CAD build for the part. Positions are in the model's coordinates, mm. Give positions to 0.01 mm unless a question says otherwise; leave off trailing zeros. Write each loop counter-clockwise with the first axis right and the second up, starting at its lowest first coordinate (ties: lowest second). Pieces come first, ordered by that corner, then holes. Notation, with made-up numbers: (-12, 38) - (6, 38) arc R18 ccw to (6, 56) - close; hole circle Ø7 at (-34, 54). An arc over 180 degrees is marked (long way). Write item = value, one per line. Start each with the question number.
```python
from build123d import *

# Parameters (mm, degrees)
F1_DEPTH = 1.6002
F3_DEPTH = 1.6012
F4_R     = 1.9939
F4_R_2   = 1.770589
F5_DEPTH = 1.6012


with BuildPart() as f1:
    # F0 (on Top) → F1 (new body)
    with BuildSketch(Plane.XY):
        with BuildLine():
            ThreePointArc((-241.3, -104.775), (-239.440128, -109.265128), (-234.95, -111.125))
            Line((-234.95, -111.125), (234.95, -111.125))
            ThreePointArc((234.95, -111.125), (239.440128, -109.265128), (241.3, -104.775))
            Line((241.3, -104.775), (241.3, 104.775))
            ThreePointArc((241.3, 104.775), (239.440128, 109.265128), (234.95, 111.125))
            Line((234.95, 111.125), (-234.95, 111.125))
            ThreePointArc((-234.95, 111.125), (-239.440128, 109.265128), (-241.3, 104.775))
            Line((-241.3, 104.775), (-241.3, -104.775))
        make_face()
    extrude(amount=-F1_DEPTH)

    # F2 (on face) → F3 (cut, through all)
    with BuildSketch(Plane.XY):
        with BuildLine():
            ThreePointArc((-222.25, -85.725), (-220.390128, -90.215128), (-215.9, -92.075))
            Line((-215.9, -92.075), (-12.7, -92.075))
            ThreePointArc((-12.7, -92.075), (-8.209872, -90.215128), (-6.35, -85.725))
            Line((-6.35, -85.725), (-6.35, 85.725))
            ThreePointArc((-6.35, 85.725), (-8.209872, 90.215128), (-12.7, 92.075))
            Line((-12.7, 92.075), (-215.9, 92.075))
            ThreePointArc((-215.9, 92.075), (-220.390128, 90.215128), (-222.25, 85.725))
            Line((-222.25, 85.725), (-222.25, -85.725))
        make_face()
        with BuildLine():
            ThreePointArc((215.9, -92.075), (220.390128, -90.215128), (222.25, -85.725))
            Line((222.25, -85.725), (222.25, 85.725))
            ThreePointArc((222.25, 85.725), (220.390128, 90.215128), (215.9, 92.075))
            Line((215.9, 92.075), (12.7, 92.075))
            ThreePointArc((12.7, 92.075), (8.209872, 90.215128), (6.35, 85.725))
            Line((6.35, 85.725), (6.35, -85.725))
            ThreePointArc((6.35, -85.725), (8.209872, -90.215128), (12.7, -92.075))
            Line((12.7, -92.075), (215.9, -92.075))
        make_face()
    extrude(amount=-F3_DEPTH, mode=Mode.SUBTRACT)

    # F4 (on face) → F5 (cut, through all)
    with BuildSketch(Plane.XY):
        with Locations((-231.3686, 103.1875)):
            Circle(F4_R)
        with Locations((0, -103.1875)):
            Circle(F4_R_2)
        with Locations((0, 103.1875)):
            Circle(F4_R)
        with Locations((233.3625, 103.1875)):
            Circle(F4_R)
        with Locations((231.819779, -103.1875)):
            Circle(F4_R)
        with Locations((-233.3625, -103.1875)):
            Circle(F4_R)
    extrude(amount=-F5_DEPTH, mode=Mode.SUBTRACT)


solid = f1.part
```
1. Wall check: line 1 along X through (y, z) = (-78, -1.3); line 2 along Y through (x, z) = (190, -0.3) (3 decimals); line 3 along X through (y, z) = (-91.5, -0.8). Give the ranges that are in metal, low to high.
2. Cut at C-C (z = -0.6). Count the separate pieces of the cut face and the enclosed holes in it, then the cut area to 3 significant figures.
3. Cut at B-B (x = -129). Give the cut face in (y, z) (3 decimals), then the cut area to 3 significant figures.
4. Cut at A-A (y = -28.5). Give the cut face in (x, z).
Output:
q1.line_1 = -241.3 to -222.25, -6.35 to 6.35, 222.25 to 241.3
q1.line_2 = -111.125 to -92.075, 92.075 to 111.125
q1.line_3 = -241.3 to -218.54, -10.06 to 10.06, 218.54 to 241.3
q2.separate_pieces = 1
q2.enclosed_holes = 8
q2.area = 27,700 mm2
q3.outline = (-111.125, -1.6) - (-92.075, -1.6) - (-92.075, 0) - (-111.125, 0) - close; (92.075, -1.6) - (111.125, -1.6) - (111.125, 0) - (92.075, 0) - close
q3.area = 61.0 mm2
q4.outline = (-241.3, -1.6) - (-222.25, -1.6) - (-222.25, 0) - (-241.3, 0) - close; (-6.35, -1.6) - (6.35, -1.6) - (6.35, 0) - (-6.35, 0) - close; (222.25, -1.6) - (241.3, -1.6) - (241.3, 0) - (222.25, 0) - close
